```python
from build123d import *

# Parameters (mm, degrees)
SKETCH_1_W           = 23
SKETCH_1_H           = 23
SKETCH_1_W_2         = 21
SKETCH_1_H_2         = 21
EXTRUDE_1_DEPTH      = 4
SKETCH_2_W           = 21
SKETCH_2_H           = 21
EXTRUDE_2_DEPTH      = 2
CUT_EXTRUDE_1_DEPTH  = 2
FILLET_2_R           = 2
FILLET_3_R           = 2
EXTRUDE_6_DEPTH      = 45
SKETCH_19_W          = 23
SKETCH_19_H          = 2
EXTRUDE_7_DEPTH      = 24
SKETCH_4_R           = 1
CUT_EXTRUDE_9_DEPTH  = 20
EXTRUDE_8_DEPTH      = 5
SKETCH_22_R          = 8.5
SKETCH_22_R_2        = 1
CUT_EXTRUDE_11_DEPTH = 5


with BuildPart() as part:
    # 草图1 → 凸台-拉伸1 (new body)
    with BuildSketch(Plane(origin=(0, 0, 0), x_dir=(1, 0, 0), z_dir=(0, 1, 0))):
        with Locations((10.5, 10.5)):
            Rectangle(SKETCH_1_W, SKETCH_1_H)
        with Locations((10.5, 10.5)):
            Rectangle(SKETCH_1_W_2, SKETCH_1_H_2, mode=Mode.SUBTRACT)
    extrude(amount=EXTRUDE_1_DEPTH)

    # 草图2 → 凸台-拉伸2 (add)
    with BuildSketch(Plane(origin=(0, 0, 0), x_dir=(1, 0, 0), z_dir=(0, 1, 0))):
        with Locations((10.5, 10.5)):
            Rectangle(SKETCH_2_W, SKETCH_2_H)
    extrude(amount=EXTRUDE_2_DEPTH)

    # 草图3 → 切除-拉伸1 (cut)
    with BuildSketch(Plane(origin=(0, 2, 0), x_dir=(1, 0, 0), z_dir=(0, 1, 0))):
        with BuildLine():
            ThreePointArc((19.5, 10.5), (10.5, 19.5), (1.5, 10.5))
            Line((1.5, 10.5), (19.5, 10.5))
        make_face()
        with BuildLine():
            Line((19.5, 10.5), (1.5, 10.5))
            ThreePointArc((1.5, 10.5), (10.5, 1.5), (19.5, 10.5))
        make_face()
    extrude(amount=-CUT_EXTRUDE_1_DEPTH, mode=Mode.SUBTRACT)

    # 圆角2
    fillet_2_edges = [part.edges().sort_by_distance(p)[0] for p in [
        (-1, 2, -22),
    ]]
    fillet(fillet_2_edges, radius=FILLET_2_R)

    # 圆角3
    fillet_3_edges = [part.edges().sort_by_distance(p)[0] for p in [
        (22, 2, -22),
    ]]
    fillet(fillet_3_edges, radius=FILLET_3_R)

    # 草图18 → 凸台-拉伸6 (add)
    with BuildSketch(Plane.XY.offset(1)):
        Polygon((-1, 0), (22, 0), (22, 10), (21, 10), (21, 1), (0, 1), (0, 10), (-1, 10), align=None)
    extrude(amount=EXTRUDE_6_DEPTH)

    # 草图19 → 凸台-拉伸7 (add)
    with BuildSketch(Plane(origin=(0, 1, 0), x_dir=(1, 0, 0), z_dir=(0, 1, 0))):
        with Locations((10.5, -45)):
            Rectangle(SKETCH_19_W, SKETCH_19_H)
    extrude(amount=EXTRUDE_7_DEPTH)

    # 草图4 → 切除-拉伸9 (cut)
    with BuildSketch(Plane(origin=(0, 2, 0), x_dir=(1, 0, 0), z_dir=(0, 1, 0))):
        with Locations(Location((2.8, 18.2, 0), (0, 0, 270))):
            Circle(SKETCH_4_R)
        with Locations(Location((2.8, 2.8, 0), (0, 0, 270))):
            Circle(SKETCH_4_R)
        with Locations(Location((18.2, 2.8, 0), (0, 0, 270))):
            Circle(SKETCH_4_R)
        with Locations(Location((18.2, 18.2, 0), (0, 0, 270))):
            Circle(SKETCH_4_R)
    extrude(amount=-CUT_EXTRUDE_9_DEPTH, mode=Mode.SUBTRACT)

    # 草图24 → 凸台-拉伸8 (add)
    with BuildSketch(Plane(origin=(0, 0, 44), x_dir=(-1, 0, 0), z_dir=(0, 0, -1))):
        Polygon((-22, 10), (-22, 25), (1, 25), (1, 10), (0, 10), (0, 24), (-21, 24), (-21, 10), align=None)
    extrude(amount=EXTRUDE_8_DEPTH)

    # 草图22 → 切除-拉伸11 (cut)
    with BuildSketch(Plane.XY.offset(46)):
        with Locations((10.5, 13.5)):
            Circle(SKETCH_22_R)
        with Locations((18.2, 21.2)):
            Circle(SKETCH_22_R_2)
        with Locations((2.8, 21.2)):
            Circle(SKETCH_22_R_2)
        with Locations((2.8, 5.8)):
            Circle(SKETCH_22_R_2)
        with Locations((18.2, 5.8)):
            Circle(SKETCH_22_R_2)
    extrude(amount=-CUT_EXTRUDE_11_DEPTH, mode=Mode.SUBTRACT)


solid = part.part
```
Input: part model. Units: mm. Frame: model coordinates. A direction names the side the tool comes from. Round coordinates to 2 decimals unless told otherwise and drop trailing zeros. Loops run counter-clockwise (first coordinate to the right, second up) from the corner with the lowest first, then second, coordinate; pieces in that order, holes last. Notation, with made-up numbers: (67.25, 33.25) -> (71.25, 33.25) arc R18 ccw to (71.25, 50.25) -> close; hole circle Ø2 at (0, -31.75). An arc over 180 degrees is marked (long way). Use one line per item in the form item = value. Start each with the question number.
Item 1: Section query A-A on x = 10.5. Return the cut outline in (y, z), then the cut area to 3 significant figures.
Item 2: Material intervals for L1, parallel to X at y = 16.75, z = 42; L2, parallel to Y at x = 10.5, z = 45; L3, parallel to Y at x = 18.2, z = 45, sorted ascending. Write a range as from..to.
Item 3: Section query D-D on y = 10.75. Return the cut outline in (x, z).
Item 4: Mould query, pull axis Y, two halves, no side actions, for faces 1 (the face through (17.224, 1.014, -3.017)), 2 (the face through (0, 7, 23)), 3 (the face through (10, 2, -1)). Classes: pulls with the +Y half, pulls with the -Y half, needs draft (parallel to the pull), parting line crosses it, or undercut.
Item 5: Section query C-C on y = 21.2. Return the cut outline in (x, z).
Item 6: Set-up query: faces 4 (the face through (21, 3, -10)), 5 (the face through (17.64, 1.01, -15.98)), 6 (the face through (9.6, 24.2, 39)), 7 (the face through (10.4, 4.7, 44)). Return all of +Z, -Z, +X, -X, +Y, -Y with unobstructed straight access to the full face (end or side cutting, diameter ignored); none if empty.
Item 7: Contact query for flat-ended pins moving along their axis: pin 1 Ø6 at (x, y) = (4.5, 20.5) entering from -Z; pin 2 Ø2 at (x, z) = (6.5, 20) entering from +Y; pin 3 Ø1.2 at (x, y) = (18.2, 5.8) entering from -Z; pin 4 Ø3 at (x, z) = (2.8, -18.2) entering from +Y. Output: stop coordinate, or through.
Item 8: Section query B-B on z = -10.5. Return the cut outline in (x, y).
Ans:
q1.outline = (0, -22) -> (4, -22) -> (4, -21) -> (2, -21) -> (2, -19.5) -> (0, -19.5) -> close; (0, -1.5) -> (2, -1.5) -> (2, 0) -> (4, 0) -> (4, 1) -> (1, 1) -> (1, 44) -> (5, 44) -> (5, 46) -> (0, 46) -> close; (22, 44) -> (24, 44) -> (24, 39) -> (25, 39) -> (25, 46) -> (22, 46) -> close
q1.area = 78.0 mm^2
q2.L1 = -1..0, 21..22
q2.L2 = 0..5, 22..25
q2.L3 = 0..4.8, 6.8..9.9, 17.1..20.2, 22.2..25
q3.outline = (-1, 39) -> (0, 39) -> (0, 44) -> (2.46, 44) -> (2.46, 46) -> (-1, 46) -> close; (18.54, 44) -> (21, 44) -> (21, 39) -> (22, 39) -> (22, 46) -> (18.54, 46) -> close
q4.face_1 = needs draft
q4.face_2 = undercut
q4.face_3 = pulls with the +Y half
q5.outline = (-1, 39) -> (0, 39) -> (0, 44) -> (1.8, 44) -> (1.8, 46) -> (-1, 46) -> close; (3.8, 44) -> (6.9, 44) -> (6.9, 46) -> (3.8, 46) -> close; (14.1, 44) -> (17.2, 44) -> (17.2, 46) -> (14.1, 46) -> close; (19.2, 44) -> (21, 44) -> (21, 39) -> (22, 39) -> (22, 46) -> (19.2, 46) -> close
q6.face_4 = +Y
q6.face_5 = +Y, -Y
q6.face_6 = -Z, +X, -X, +Y
q6.face_7 = none
q7.pin_1 = 44
q7.pin_2 = 1
q7.pin_3 = through
q7.pin_4 = 2
q8.outline = (-1, 0) -> (1.5, 0) -> (1.5, 2) -> (0, 2) -> (0, 4) -> (-1, 4) -> close; (19.5, 0) -> (22, 0) -> (22, 4) -> (21, 4) -> (21, 2) -> (19.5, 2) -> close
